from build123d import *

# Parameters (mm, degrees)
F1_DEPTH = 1574.8
F3_DEPTH = 19.05
F4_R     = 9.525
F5_DEPTH = 43.942
F6_R     = 9.525
F7_DEPTH = 25.4


with BuildPart() as f1:
    # F0 (on Front) → F1 (new body)
    with BuildSketch(Plane.XZ):
        with BuildLine():
            Line((76.073, 76.073), (-76.073, 76.073))
            Line((-76.073, 76.073), (-76.073, 69.469))
            Line((-76.073, 69.469), (-9.271, 69.469))
            ThreePointArc((-9.271, 69.469), (-4.780872, 67.609128), (-2.921, 63.119))
            Line((-2.921, 63.119), (-2.921, -63.119))
            ThreePointArc((-2.921, -63.119), (-4.780872, -67.609128), (-9.271, -69.469))
            Line((-9.271, -69.469), (-76.073, -69.469))
            Line((-76.073, -69.469), (-76.073, -76.073))
            Line((-76.073, -76.073), (76.073, -76.073))
            Line((76.073, -76.073), (76.073, -69.469))
            Line((76.073, -69.469), (9.271, -69.469))
            ThreePointArc((9.271, -69.469), (4.780872, -67.609128), (2.921, -63.119))
            Line((2.921, -63.119), (2.921, 63.119))
            ThreePointArc((2.921, 63.119), (4.780872, 67.609128), (9.271, 69.469))
            Line((9.271, 69.469), (76.073, 69.469))
            Line((76.073, 69.469), (76.073, 76.073))
        make_face()
    extrude(amount=F1_DEPTH)

    # F2 (on face) → F3 (join)
    with BuildSketch(Plane.XZ.offset(1574.8)):
        with BuildLine():
            Line((-9.271, 69.469), (-76.073, 69.469))
            Line((-76.073, 69.469), (-76.073, -69.469))
            Line((-76.073, -69.469), (-9.271, -69.469))
            ThreePointArc((-9.271, -69.469), (-4.780872, -67.609128), (-2.921, -63.119))
            Line((-2.921, -63.119), (-2.921, 63.119))
            ThreePointArc((-2.921, 63.119), (-4.780872, 67.609128), (-9.271, 69.469))
        make_face()
        with BuildLine():
            Line((76.073, 76.073), (-76.073, 76.073))
            Line((-76.073, 76.073), (-76.073, 69.469))
            Line((-76.073, 69.469), (-9.271, 69.469))
            ThreePointArc((-9.271, 69.469), (-4.780872, 67.609128), (-2.921, 63.119))
            Line((-2.921, 63.119), (-2.921, -63.119))
            ThreePointArc((-2.921, -63.119), (-4.780872, -67.609128), (-9.271, -69.469))
            Line((-9.271, -69.469), (-76.073, -69.469))
            Line((-76.073, -69.469), (-76.073, -76.073))
            Line((-76.073, -76.073), (76.073, -76.073))
            Line((76.073, -76.073), (76.073, -69.469))
            Line((76.073, -69.469), (9.271, -69.469))
            ThreePointArc((9.271, -69.469), (4.780872, -67.609128), (2.921, -63.119))
            Line((2.921, -63.119), (2.921, 63.119))
            ThreePointArc((2.921, 63.119), (4.780872, 67.609128), (9.271, 69.469))
            Line((9.271, 69.469), (76.073, 69.469))
            Line((76.073, 69.469), (76.073, 76.073))
        make_face()
        with BuildLine():
            Line((76.073, -69.469), (76.073, 69.469))
            Line((76.073, 69.469), (9.271, 69.469))
            ThreePointArc((9.271, 69.469), (4.780872, 67.609128), (2.921, 63.119))
            Line((2.921, 63.119), (2.921, -63.119))
            ThreePointArc((2.921, -63.119), (4.780872, -67.609128), (9.271, -69.469))
            Line((9.271, -69.469), (76.073, -69.469))
        make_face()
    extrude(amount=F3_DEPTH)

    # F4 (on face) → F5 (cut)
    with BuildSketch(Plane.XZ.offset(1593.85)):
        with Locations((-37.973, -44.323)):
            Circle(F4_R)
        with Locations((37.973, -44.323)):
            Circle(F4_R)
    extrude(amount=-F5_DEPTH, mode=Mode.SUBTRACT)

    # F6 (on face) → F7 (cut)
    with BuildSketch(Plane(origin=(0, 0, -76.073), x_dir=(1, 0, 0), z_dir=(0, 0, -1))):
        with Locations((-37.973, 812.8)):
            Circle(F6_R)
        with Locations((37.973, 812.8)):
            Circle(F6_R)
        with Locations((-37.973, 635)):
            Circle(F6_R)
        with Locations((37.973, 635)):
            Circle(F6_R)
        with Locations((-37.973, 352.425)):
            Circle(F6_R)
        with Locations((37.973, 352.425)):
            Circle(F6_R)
        with Locations((-37.973, 203.2)):
            Circle(F6_R)
        with Locations((37.973, 203.2)):
            Circle(F6_R)
        with Locations((-37.973, 53.975)):
            Circle(F6_R)
        with Locations((37.973, 53.975)):
            Circle(F6_R)
    extrude(amount=-F7_DEPTH, mode=Mode.SUBTRACT)


solid = f1.part
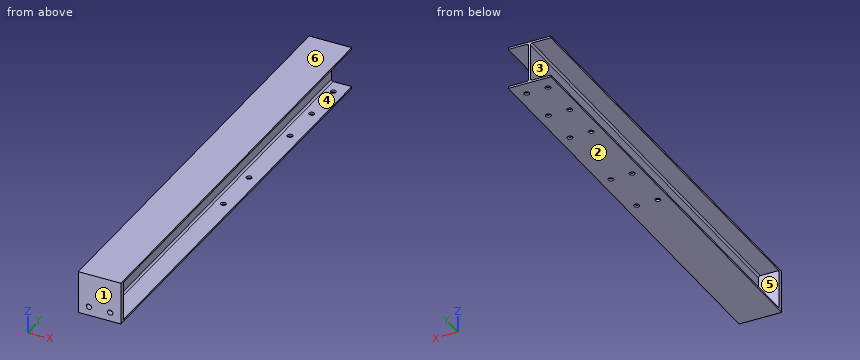
Here's how the part is built. I have some questions about the finished solid (model axes, mm). Face numbers are marked on the shaded views. A direction names the side the tool comes from. Coordinates: 2 decimals unless noted, no trailing zeros. Write each loop counter-clockwise with the first axis right and the second up, starting at its lowest first coordinate (ties: lowest second). Pieces come first, ordered by that corner, then holes.
Item 1: If we mould it in two halves opening along Z, with no side actions, what happens to the marked faces 1, 2 and 3? For each: +Z half, -Z half, draft (parallel to the pull), parting line (faces both ways), or undercut.
Item 2: On a 3-axis mill with a long thin cutter (end or side, diameter ignored), from which of +Z, -Z, +X, -X, +Y, -Y can I reach the whole of each face in a straight line? I mean the marked faces 4, 5 and 6. Say none if no direction works.
Item 3: I want a section at A-A on y = -1037. Write out the boundary of the cut face in (x, z), and give its area (3 significant figures).
Item 4: If I drill on line 1 (X direction, y = -635, z = -72); line 2 (Z direction, x = -16, y = -1468.5); line 3 (X direction, y = -863, z = 5.5), over which ranges is the centre line in solid material (lowest first)?
Item 5: Will these pins go through, and if not, where does the flat tip stop? pin 1 (1.5 mm diameter, centred on y = -559, z = -57, fed in from +X); pin 2 (17 mm diameter, centred on x = -37.973, z = -44.323, fed in from +Y); pin 3 (22 mm diameter, centred on x = 37.973, z = -44.323, fed in from +Y).
Item 6: I want a section at B-B on z = 21.5. Write out the boundary of the cut face in (x, y), and give its area (3 significant figures).
Findings below:
1. face 1: draft
1. face 2: -Z half
1. face 3: undercut
2. face 4: +X, +Y
2. face 5: -X, +Y
2. face 6: +Z, +X, -X, +Y, -Y
3. outline: (-76.07, -76.07) - (76.07, -76.07) - (76.07, -69.47) - (9.27, -69.47) arc R6.35 cw to (2.92, -63.12) - (2.92, 63.12) arc R6.35 cw to (9.27, 69.47) - (76.07, 69.47) - (76.07, 76.07) - (-76.07, 76.07) - (-76.07, 69.47) - (-9.27, 69.47) arc R6.35 cw to (-2.92, 63.12) - (-2.92, -63.12) arc R6.35 cw to (-9.27, -69.47) - (-76.07, -69.47) - close
3. area: 2,860 mm2
4. line 1: x = -76.07 to -47.5, -28.45 to 28.45, 47.5 to 76.07
4. line 2: z = -76.07 to -69.47, 69.47 to 76.07
4. line 3: x = -2.92 to 2.92
5. pin 1: stops at x = 2.92
5. pin 2: passes through
5. pin 3: stops at y = -1574.8
6. outline: (-76.07, -1593.85) - (76.07, -1593.85) - (76.07, -1574.8) - (2.92, -1574.8) - (2.92, 0) - (-2.92, 0) - (-2.92, -1574.8) - (-76.07, -1574.8) - close
6. area: 12,100 mm2
